```python
from build123d import *
from build123d.topology import SkipClean

# Parameters (mm, degrees)
EXTRUDE_1_DEPTH      = 17
EXTRUDE_1_DEPTH_BACK = 17
SKETCH_1_R           = 3.5
EXTRUDE_2_DEPTH      = 13
CUT_EXTRUDE_1_REACH  = 32.615
SKETCH_5_R           = 2


with BuildPart() as part:
    # Sketch 1 → Extrude 1 (new, two sides: drawn at the far end of the back side and taken through both)
    with BuildSketch(Plane(origin=(0, 0, 0), x_dir=(1, 0, 0), z_dir=(0, 1, 0)).offset(-EXTRUDE_1_DEPTH_BACK)):
        with Locations(Location((0, 0, 0), (0, 0, 270))):
            Circle(SKETCH_1_R)
    extrude(amount=EXTRUDE_1_DEPTH + EXTRUDE_1_DEPTH_BACK)

    # Sketch 2 → Extrude 2 (add)
    with BuildSketch(Plane.XZ.offset(17)):
        with BuildLine():
            Line((3.16227766, 1.5), (-3.16227766, 1.5))
            ThreePointArc((-3.16227766, 1.5), (-3.5, 0), (-3.16227766, -1.5))
            Line((-3.16227766, -1.5), (3.16227766, -1.5))
            ThreePointArc((3.16227766, -1.5), (3.414525722, -0.768774411), (3.5, 0))
            ThreePointArc((3.5, 0), (3.414525722, 0.768774411), (3.16227766, 1.5))
        make_face()
    extrude_2 = extrude(amount=EXTRUDE_2_DEPTH)

    # Sketch 5 → Cut-Extrude 1 (cut, up to next)
    with BuildSketch(Plane(origin=(0, 0, -1.5), x_dir=(-1, 0, 0), z_dir=(0, 0, -1)), mode=Mode.PRIVATE) as cut_extrude_1_sk1:
        with Locations((0, -26)):
            Circle(SKETCH_5_R)
    cut_extrude_1_tool1 = extrude(cut_extrude_1_sk1.sketch, amount=-CUT_EXTRUDE_1_REACH, mode=Mode.PRIVATE) & part.part
    cut_extrude_1 = cut_extrude_1_tool1.solids().sort_by_distance((0, -26, -1.5))[0]
    add(cut_extrude_1, mode=Mode.SUBTRACT)

    # Mirror 2: Extrude 2, Cut-Extrude 1 across plane
    with SkipClean():  # the faces are left unmerged after this step: merging them gives an invalid solid
        add(extrude_2.mirror(Plane.ZX))
        add(cut_extrude_1.mirror(Plane.ZX), mode=Mode.SUBTRACT)


solid = part.part
```
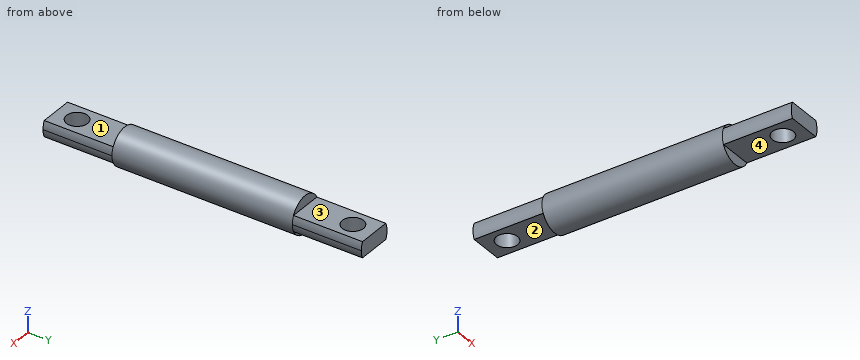
The listing builds one solid part. Answer for the finished solid, in the listing's coordinates (mm). Face numbers are marked on the shaded views. A direction names the side the tool comes from. Give positions to 0.01 mm unless a question says otherwise; leave off trailing zeros. Loops run counter-clockwise (first coordinate to the right, second up) from the corner with the lowest first, then second, coordinate; pieces in that order, holes last. Notation, with made-up numbers: M 66.5,55.5 L 75.5,55.5 A17 ccw 75.5,70.5 Z; hole C -14.75,7 d5. An arc over 180 degrees is marked long. One line per item, written item: value.
Q1. Find the intervals of material crossed by line 1 (Y direction, x = 0, z = 0.55); line 2 (Y direction, x = 2, z = 1.75); line 3 (X direction, y = 26, z = -1), in increasing order. Write a range as from..to.
Working result:
line 1: y = -30..-28, -24..24, 28..30
line 2: y = -17..17
line 3: x = -3.35..-2, 2..3.35
Q2. A cutting plane is placed at B-B on x = 0. Determine the outline of the cut face in (y, z), then the cut area to 3 significant figures.
Working result:
outline: M -30,-1.5 L -28,-1.5 L -28,1.5 L -30,1.5 Z; M -24,-1.5 L -17,-1.5 L -17,-3.5 L 17,-3.5 L 17,-1.5 L 24,-1.5 L 24,1.5 L 17,1.5 L 17,3.5 L -17,3.5 L -17,1.5 L -24,1.5 Z; M 28,-1.5 L 30,-1.5 L 30,1.5 L 28,1.5 Z
area: 292 mm^2
Q3. A cutting plane is placed at C-C on z = 0.5. Determine the outline of the cut face in (x, y), then the cut area to 3 significant figures.
Working result:
outline: M -3.46,-30 L 3.46,-30 L 3.46,30 L -3.46,30 Z; hole C 0,-26 d4; hole C 0,26 d4
area: 391 mm^2
Q4. A cutting plane is placed at A-A on y = 26. Determine the outline of the cut face in (x, z), then the cut area to 3 significant figures.
Working result:
outline: M -3.16,-1.5 L -2,-1.5 L -2,1.5 L -3.16,1.5 A3.5 ccw Z; M 2,-1.5 L 3.16,-1.5 A3.5 ccw 3.16,1.5 L 2,1.5 Z
area: 8.34 mm^2
Q5. A cutting plane is placed at D-D on y = 18. Determine the outline of the cut face in (x, z).
Working result:
outline: M -3.16,-1.5 L 3.16,-1.5 A3.5 ccw 3.16,1.5 L -3.16,1.5 A3.5 ccw Z
Q6. Flat-ended cylindrical pins translate along their axes: P1, Ø1.5, axis at x = 1, y = -15, coming from the -Z side; P2, Ø3, axis at x = -1, z = 2.5, coming from the +Y side; P3, Ø1.9, axis at x = 0, y = -24.5, coming from the +Z side; P4, Ø0.6, axis at x = -0.5, z = 2, coming from the +Y side. Find the tip coordinate at first contact, or state that the pin passes through.
Working result:
P1: stops at z = -3.49
P2: stops at y = 30
P3: stops at z = 1.5
P4: stops at y = 17
Q7. For the marked faces 1, 2, 3 and 4, determine the directions among +Z, -Z, +X, -X, +Y, -Y from which every point of the face is accessible in a straight line to the end or side of a thin tool.
Working result:
face 1: +Z, +X, -X, -Y
face 2: -Z, +X, -X, +Y
face 3: +Z, +X, -X, +Y
face 4: -Z, +X, -X, -Y
